Verification items for the finished model (mm, model axes). A direction names the side the tool comes from. Give positions to 0.01 mm unless a question says otherwise; leave off trailing zeros. Loops run counter-clockwise (first coordinate to the right, second up) from the corner with the lowest first, then second, coordinate; pieces in that order, holes last. Notation, with made-up numbers: (21.5, 81.25) - (26.5, 81.25) arc R6 ccw to (26.5, 85.25) - close; hole circle Ø8 at (54.5, 73). An arc over 180 degrees is marked (long way). One line per question, with ' | ' between items. Start each with the question number.
1. Mould release check, pull along Y, two halves, no side actions. Record for faces 1 (the face through (12.32, 2.64, 119.97)), 2 (the face through (5, -2, 44)), 3 (the face through (12, 120, -15)): +Y half, -Y half, draft (parallel to the pull), parting line (faces both ways), or undercut.
2. Thickness scan on line 1 along Y through (x, z) = (11.25, -11.5); line 2 along X through (y, z) = (6.5, 114.5); line 3 along Y through (x, z) = (16.5, 77). Record the ranges inside material, lowest first. Write a range as from..to.
3. Section check B-B, the plane x = 17.75. Enter the section's corners in (y, z), then the cut area to 3 significant figures.
4. Section check D-D, the plane z = 46. Enter the section's corners in (x, y), then the cut area to 3 significant figures.
5. Section check C-C, the plane z = 14. Enter the section's corners in (x, y), then the cut area to 3 significant figures.
6. Section check A-A, the plane y = 0. Enter the section's corners in (x, z), then the cut area to 3 significant figures.
7. Tool access check on faces 4 (the face through (14.86, -2.529, 114.972)), 5 (the face through (2, -26, -2)), 6 (the face through (25, -27, 112)). Record the directions out of +Z, -Z, +X, -X, +Y, -Y that give a thin tool (end or side, any length) a straight path to the whole face; none if there is none.
8. Depth check by flat-ended pin: pin 1 Ø2 at (x, z) = (19, 34.5) entering from +Y; pin 2 Ø10 at (y, z) = (-94, 55.5) entering from +X; pin 3 Ø10 at (x, y) = (9.5, -33) entering from +Z. Enter the tip coordinate at first touch or a pass-through.
from build123d import *

# Parameters (mm, degrees)
F1_DEPTH = 5
F2_DEPTH = 25


with BuildPart() as f1:
    # F0 (on Right) → F1 (new body)
    with BuildSketch(Plane.YZ):
        with BuildLine():
            Line((115, -30), (115, 0))
            ThreePointArc((115, 0), (0, 115), (-115, 0))
            Line((-115, 0), (-115, -30))
            Line((-115, -30), (-26, -30))
            Line((-26, -30), (-26, 26))
            Line((-26, 26), (0, 26))
            Line((0, 26), (26, 26))
            Line((26, 26), (26, -30))
            Line((26, -30), (115, -30))
        make_face()
    extrude(amount=F1_DEPTH)

    # F0 (on Right) → F2 (join)
    with BuildSketch(Plane.YZ):
        with BuildLine():
            ThreePointArc((-115, 0), (0, 115), (115, 0))
            Line((115, 0), (115, -30))
            Line((115, -30), (116.1895, -30))
            Line((116.1895, -30), (120, -30))
            Line((120, -30), (120, 0))
            ThreePointArc((120, 0), (0, 120), (-120, 0))
            Line((-120, 0), (-120, -30))
            Line((-120, -30), (-115, -30))
            Line((-115, -30), (-115, 0))
        make_face()
    extrude(amount=F2_DEPTH)


solid = f1.part
Results list:
1) face 1: parting line | face 2: undercut | face 3: +Y half
2) line 1: -120..-115, 115..120 | line 2: 0..5 | line 3: -92.04..-85.42, 85.42..92.04
3) outline: (-120, -30) - (-115, -30) - (-115, 0) arc R115 cw to (115, 0) - (115, -30) - (120, -30) - (120, 0) arc R120 ccw to (-120, 0) - close | area: 2,150 mm²
4) outline: (0, -110.83) - (25, -110.83) - (25, -105.4) - (5, -105.4) - (5, 105.4) - (25, 105.4) - (25, 110.83) - (0, 110.83) - close | area: 1,330 mm²
5) outline: (0, -119.18) - (25, -119.18) - (25, -114.14) - (5, -114.14) - (5, -26) - (0, -26) - close; (0, 26) - (5, 26) - (5, 114.14) - (25, 114.14) - (25, 119.18) - (0, 119.18) - close | area: 1,130 mm²
6) outline: (0, 26) - (5, 26) - (5, 115) - (25, 115) - (25, 120) - (0, 120) - close | area: 570 mm²
7) face 4: -Z, +X | face 5: -Z, +X, -X | face 6: +Z, -Z, +X, +Y, -Y
8) pin 1: y = 115.23 | pin 2: x = 5 | pin 3: z = 116.69
